Design review of the part built by this model. Coordinates are the model's own, in mm. Face numbers are marked on the shaded views. A direction names the side the tool comes from. Give positions to 0.01 mm unless a question says otherwise; leave off trailing zeros. Write each loop counter-clockwise with the first axis right and the second up, starting at its lowest first coordinate (ties: lowest second). Pieces come first, ordered by that corner, then holes. Notation, with made-up numbers: M 7.5,70 L 19.5,70 A17 cw 19.5,98 Z; hole C 33.25,78.5 d10. An arc over 180 degrees is marked long. Answer in a Markdown table with one row per item.
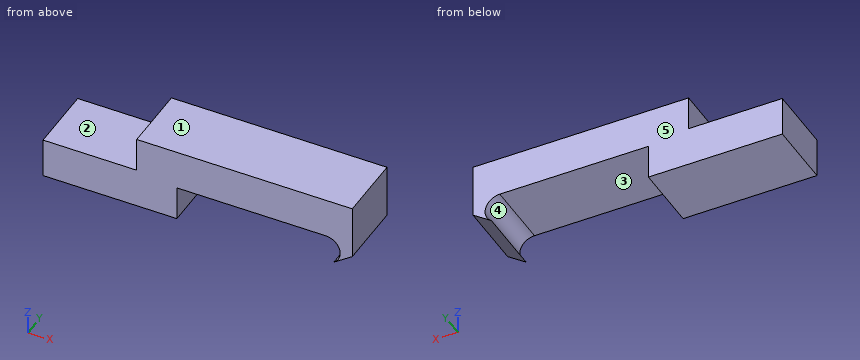
```python
from build123d import *

# Parameters (mm, degrees)
F1_DEPTH = 25


with BuildPart() as f1:
    # F0 (on Front) → F1 (new body)
    with BuildSketch(Plane.XZ):
        with BuildLine():
            Line((-50, 15), (-50, 0))
            Line((-50, 0), (0, 0))
            Line((0, 0), (0, 13))
            Line((0, 13), (55.5, 13))
            ThreePointArc((55.5, 13), (60.745443, 9.153882), (58.65467, 2.994664))
            Line((58.65467, 2.994664), (65.5, 7.787815))
            Line((65.5, 7.787815), (65.5, 28))
            Line((65.5, 28), (-15, 28))
            Line((-15, 28), (-15, 15))
            Line((-15, 15), (-50, 15))
        make_face()
    extrude(amount=F1_DEPTH)


solid = f1.part
```
1) Add section C-C (x = -41). Write out the cut boundary in (y, z), and give its area (3 significant figures).
Geometry says:
| item | result |
|---|---|
| outline | M -25,0 L 0,0 L 0,15 L -25,15 Z |
| area | 375 mm^2 |
2) To check wall thickness, follow probe 1 along Z at (x, y) = (-39.5, -1.75); probe 2 along X at (y, z) = (-22.5, 2.75); probe 3 along Z at (x, y) = (10, -12.25). State the ranges of each line that lie inside material, in increasing order. Write a range as [from, to].
Geometry says:
| item | result |
|---|---|
| probe 1 | [0, 15] |
| probe 2 | [-50, 0] |
| probe 3 | [13, 28] |
3) Add section A-A (y = -13.5). Write out the cut boundary in (x, z).
Geometry says:
| item | result |
|---|---|
| outline | M -50,0 L 0,0 L 0,13 L 55.5,13 A5.5 cw 58.65,2.99 L 65.5,7.79 L 65.5,28 L -15,28 L -15,15 L -50,15 Z |
4) The part is to be moulded in two halves that separate along Z. For the marked faces 3, 4 and 5, say which applies: released by +Z, released by -Z, zero draft, split by the parting line, or undercut.
Geometry says:
| item | result |
|---|---|
| face 3 | released by -Z |
| face 4 | undercut |
| face 5 | zero draft |
5) Add section B-B (z = 25). Write out the cut boundary in (x, y), and give its area (3 significant figures).
Geometry says:
| item | result |
|---|---|
| outline | M -15,-25 L 65.5,-25 L 65.5,0 L -15,0 Z |
| area | 2,010 mm^2 |
6) For the marked faces 1 and 2, list the 3-axis set-ups (+Z, -Z, +X, -X, +Y, -Y) from which the entire face can be reached by the end or side of a thin tool; tool diameter is ignored.
Geometry says:
| item | result |
|---|---|
| face 1 | +Z, +X, -X, +Y, -Y |
| face 2 | +Z, -X, +Y, -Y |
7) Insertion check: P1, Ø8, axis at x = 7, y = -17.5, coming from the -Z side; P2, Ø10.5, axis at y = -12, z = 24.5, coming from the -X side. Each pin has a flat end and moves straight along its axis. Give the tip position at first contact, or say it passes through.
Geometry says:
| item | result |
|---|---|
| P1 | z = 13 |
| P2 | x = -15 |
